```python
from build123d import *

# Parameters (mm, degrees)
SKETCH1_W           = 51.3
SKETCH1_H           = 5
BOSS_EXTRUDE1_DEPTH = 13.5
SKETCH2_W           = 0.64
SKETCH2_H           = 0.64
BOSS_EXTRUDE2_DEPTH = 3


with BuildPart() as part:
    # Sketch1 → Boss-Extrude1 (new body)
    with BuildSketch(Plane(origin=(0, 0, 0), x_dir=(1, 0, 0), z_dir=(0, 1, 0))):
        Rectangle(SKETCH1_W, SKETCH1_H)
    extrude(amount=BOSS_EXTRUDE1_DEPTH)

    # Sketch2 → Boss-Extrude2 (add)
    with BuildSketch(Plane.XZ):
        with Locations((-21.59, 1.27)):
            Rectangle(SKETCH2_W, SKETCH2_H)
        with Locations((-24.13, 1.27)):
            Rectangle(SKETCH2_W, SKETCH2_H)
        with Locations((-19.05, 1.27)):
            Rectangle(SKETCH2_W, SKETCH2_H)
        with Locations((-16.51, 1.27)):
            Rectangle(SKETCH2_W, SKETCH2_H)
        with Locations((-13.97, 1.27)):
            Rectangle(SKETCH2_W, SKETCH2_H)
        with Locations((-11.43, 1.27)):
            Rectangle(SKETCH2_W, SKETCH2_H)
        with Locations((-8.89, 1.27)):
            Rectangle(SKETCH2_W, SKETCH2_H)
        with Locations((-6.35, 1.27)):
            Rectangle(SKETCH2_W, SKETCH2_H)
        with Locations((-3.81, 1.27)):
            Rectangle(SKETCH2_W, SKETCH2_H)
        with Locations((-1.27, 1.27)):
            Rectangle(SKETCH2_W, SKETCH2_H)
        with Locations((24.13, 1.27)):
            Rectangle(SKETCH2_W, SKETCH2_H)
        with Locations((1.27, 1.27)):
            Rectangle(SKETCH2_W, SKETCH2_H)
        with Locations((3.81, 1.27)):
            Rectangle(SKETCH2_W, SKETCH2_H)
        with Locations((6.35, 1.27)):
            Rectangle(SKETCH2_W, SKETCH2_H)
        with Locations((8.89, 1.27)):
            Rectangle(SKETCH2_W, SKETCH2_H)
        with Locations((11.43, 1.27)):
            Rectangle(SKETCH2_W, SKETCH2_H)
        with Locations((13.97, 1.27)):
            Rectangle(SKETCH2_W, SKETCH2_H)
        with Locations((16.51, 1.27)):
            Rectangle(SKETCH2_W, SKETCH2_H)
        with Locations((19.05, 1.27)):
            Rectangle(SKETCH2_W, SKETCH2_H)
        with Locations((21.59, 1.27)):
            Rectangle(SKETCH2_W, SKETCH2_H)
        with Locations((21.59, -1.27)):
            Rectangle(SKETCH2_W, SKETCH2_H)
        with Locations((19.05, -1.27)):
            Rectangle(SKETCH2_W, SKETCH2_H)
        with Locations((16.51, -1.27)):
            Rectangle(SKETCH2_W, SKETCH2_H)
        with Locations((13.97, -1.27)):
            Rectangle(SKETCH2_W, SKETCH2_H)
        with Locations((11.43, -1.27)):
            Rectangle(SKETCH2_W, SKETCH2_H)
        with Locations((8.89, -1.27)):
            Rectangle(SKETCH2_W, SKETCH2_H)
        with Locations((6.35, -1.27)):
            Rectangle(SKETCH2_W, SKETCH2_H)
        with Locations((3.81, -1.27)):
            Rectangle(SKETCH2_W, SKETCH2_H)
        with Locations((1.27, -1.27)):
            Rectangle(SKETCH2_W, SKETCH2_H)
        with Locations((24.13, -1.27)):
            Rectangle(SKETCH2_W, SKETCH2_H)
        with Locations((-1.27, -1.27)):
            Rectangle(SKETCH2_W, SKETCH2_H)
        with Locations((-3.81, -1.27)):
            Rectangle(SKETCH2_W, SKETCH2_H)
        with Locations((-6.35, -1.27)):
            Rectangle(SKETCH2_W, SKETCH2_H)
        with Locations((-8.89, -1.27)):
            Rectangle(SKETCH2_W, SKETCH2_H)
        with Locations((-11.43, -1.27)):
            Rectangle(SKETCH2_W, SKETCH2_H)
        with Locations((-13.97, -1.27)):
            Rectangle(SKETCH2_W, SKETCH2_H)
        with Locations((-16.51, -1.27)):
            Rectangle(SKETCH2_W, SKETCH2_H)
        with Locations((-19.05, -1.27)):
            Rectangle(SKETCH2_W, SKETCH2_H)
        with Locations((-21.59, -1.27)):
            Rectangle(SKETCH2_W, SKETCH2_H)
        with Locations((-24.13, -1.27)):
            Rectangle(SKETCH2_W, SKETCH2_H)
    extrude(amount=BOSS_EXTRUDE2_DEPTH)


solid = part.part
```
CAD build for the part. Positions are in the model's coordinates, mm. Coordinates: 2 decimals unless noted, no trailing zeros. Order: outer loops, then holes, each group sorted by start corner. A loop starts at its lowest first (then second) coordinate and runs counter-clockwise, first axis right, second up.
(1) Drill centre line: L1, parallel to Y at x = -20.5, z = 0.7. Where is it in solid material? Low to high.
Solution:
L1: y = 0 to 13.5
(2) Saw through at B-B, the plane x = -17.5. Write the cut outline in (y, z).
Solution:
outline: (0, -2.5) - (13.5, -2.5) - (13.5, 2.5) - (0, 2.5) - close
(3) Pin check, flat tips, straight feed: pin 1 Ø0.7 at (y, z) = (-1, -1.5) entering from -X; pin 2 Ø0.5 at (x, y) = (-6.5, -1) entering from +Z; pin 3 Ø1.5 at (y, z) = (-1, -1) entering from +X. Stop position of each tip, or through.
Solution:
pin 1: stops at x = -24.45
pin 2: stops at z = 1.59
pin 3: stops at x = 24.45
(4) Saw through at A-A, the plane y = -1.25. Count the separate pieces of the cut face and the enclosed holes in it, and give its area (3 significant figures).
Solution:
separate pieces: 40
enclosed holes: 0
area: 16.4 mm2
